Geometry check sheet. Reference: drawing and pictorial views, mm from the part's lowest x, y, z. Coordinates: 2 decimals unless noted, no trailing zeros. Write each loop counter-clockwise with the first axis right and the second up, starting at its lowest first coordinate (ties: lowest second). Pieces come first, ordered by that corner, then holes. Notation, with made-up numbers: (16.25, 66) - (23.25, 66) arc R31 cw to (23.25, 96) - close; hole circle Ø2 at (41, -1). An arc over 180 degrees is marked (long way). Answer as a JSON object with one key per item and string values. Group by question number.
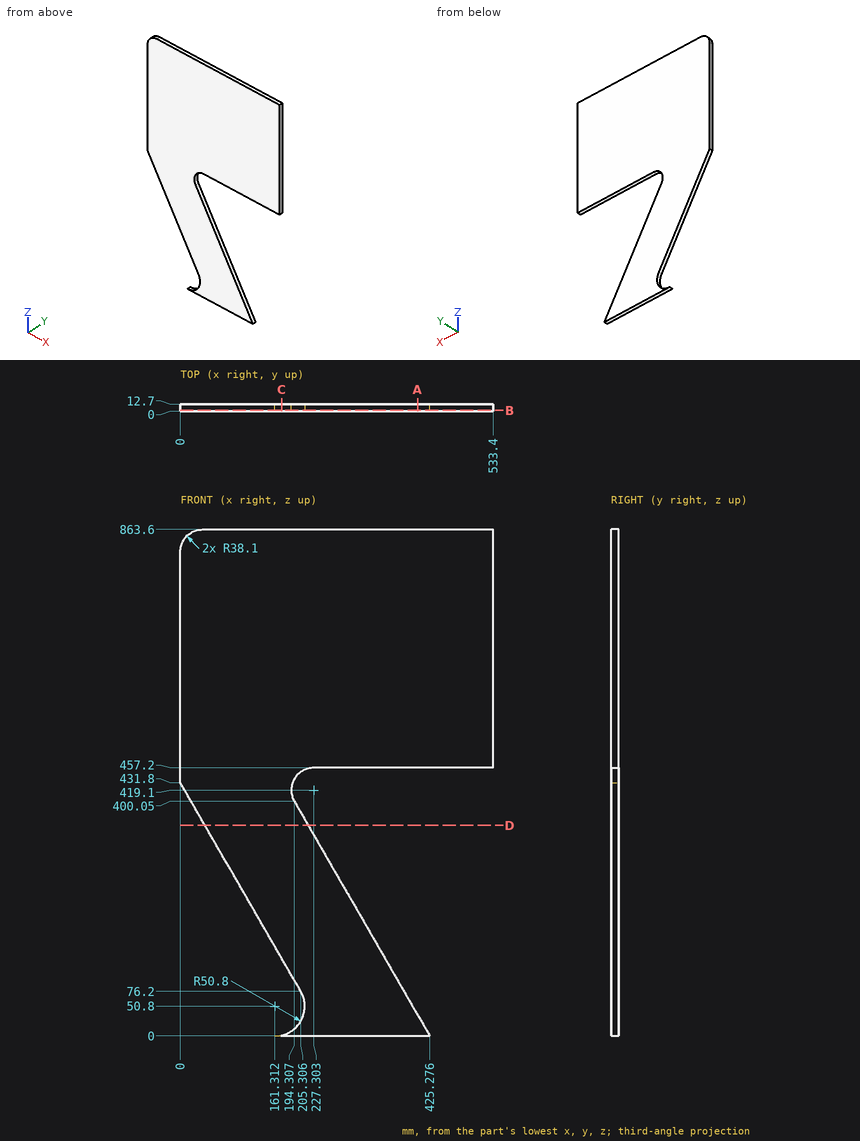
(1) Section check C-C (x = 172.5). Record the cut outline in (y, z).
(2) Section check D-D (z = 359). Record the cut outline in (x, y), and give its area (4 significant figures).
(3) Section check A-A (x = 404.5). Record the cut outline in (y, z) (1 decimal).
(4) Material ranges on L1, parallel to Z at x = 465, y = 10; L2, parallel to Z at x = 344.5, y = 11.75; L3, parallel to Z at x = 399.5, y = 5.75 (1 decimal), recorded low to high. Write a range as [from, to].
(5) Section check B-B (y = 2). Record the cut outline in (x, z), and give its area (3 significant figures).
Conclusion:
{
 "1": {"outline": "(0, 0) - (12.7, 0) - (12.7, 1.25) - (0, 1.25) - close; (0, 133.02) - (12.7, 133.02) - (12.7, 863.6) - (0, 863.6) - close"},
 "2": {"outline": "(42.03, 0) - (218.01, 0) - (218.01, 12.7) - (42.03, 12.7) - close", "area": "2,235 mm^2"},
 "3": {"outline": "(0, 0) - (12.7, 0) - (12.7, 36) - (0, 36) - close; (0, 457.2) - (12.7, 457.2) - (12.7, 863.6) - (0, 863.6) - close"},
 "4": {"L1": "z = [457.2, 863.6]", "L2": "z = [0, 139.91], [457.2, 863.6]", "L3": "z = [0, 44.6], [457.2, 863.6]"},
 "5": {"outline": "(0, 431.8) - (205.31, 76.2) arc R50.8 cw to (161.31, 0) - (425.28, 0) - (194.31, 400.05) arc R38.1 cw to (227.3, 457.2) - (533.4, 457.2) - (533.4, 863.6) - (38.1, 863.6) arc R38.1 ccw to (0, 825.5) - close", "area": "299,000 mm^2"}
}
